The listing builds one solid part. Answer for the finished solid, in the listing's coordinates (mm). Face numbers are marked on the shaded views. A direction names the side the tool comes from. Coordinates: 2 decimals unless noted, no trailing zeros. Loops run counter-clockwise (first coordinate to the right, second up) from the corner with the lowest first, then second, coordinate; pieces in that order, holes last. Notation, with made-up numbers: M -22.5,18.5 L -13.5,18.5 A11 cw -13.5,33.5 Z; hole C 88,-37.75 d8. An arc over 180 degrees is marked long. Answer as CSV lines item,"result". Start each with the question number.
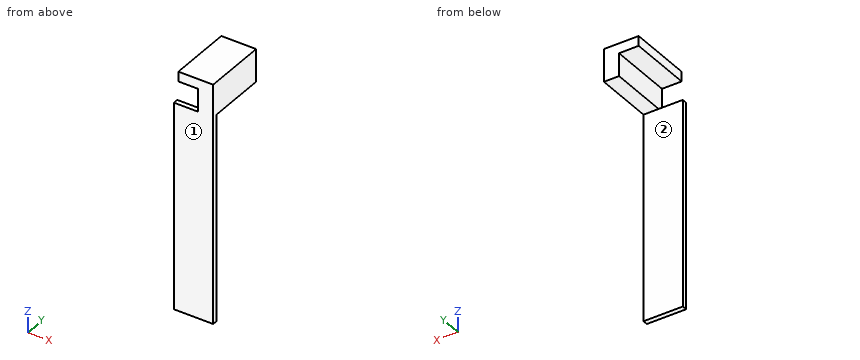
```python
from build123d import *

# Parameters (mm, degrees)
SCHIZZO1_W                   = 8
SCHIZZO1_H                   = 42.07
ESTRUSIONE_ESTRUSIONE1_DEPTH = 1
SCHIZZO2_W                   = 3.084803914
SCHIZZO2_H                   = 1
ESTRUSIONE_ESTRUSIONE2_DEPTH = 4.66
SCHIZZO3_W                   = 3.084803914
SCHIZZO3_H                   = 1
ESTRUSIONE_ESTRUSIONE3_DEPTH = 2
SCHIZZO4_W                   = 2.003143521
SCHIZZO4_H                   = 1
ESTRUSIONE_ESTRUSIONE4_DEPTH = 4
SCHIZZO5_W                   = 7.084803914
SCHIZZO5_H                   = 2.003143521
ESTRUSIONE_ESTRUSIONE5_DEPTH = 12
SCHIZZO7_W                   = 3.084803914
SCHIZZO7_H                   = 4.656856479
ESTRUSIONE_ESTRUSIONE7_DEPTH = 12


with BuildPart() as part:
    # Schizzo1 → Estrusione-Estrusione1 (new body)
    with BuildSketch(Plane(origin=(0, 0, 0), x_dir=(1, 0, 0), z_dir=(0, 1, 0))):
        with Locations((4, 21.035)):
            Rectangle(SCHIZZO1_W, SCHIZZO1_H)
    extrude(amount=ESTRUSIONE_ESTRUSIONE1_DEPTH)

    # Schizzo2 → Estrusione-Estrusione2 (add)
    with BuildSketch(Plane.XY):
        with Locations((6.457598043, 0.5)):
            Rectangle(SCHIZZO2_W, SCHIZZO2_H)
    extrude(amount=ESTRUSIONE_ESTRUSIONE2_DEPTH)

    # Schizzo3 → Estrusione-Estrusione3 (add)
    with BuildSketch(Plane.XY.offset(4.66)):
        with Locations((6.457598043, 0.5)):
            Rectangle(SCHIZZO3_W, SCHIZZO3_H)
    extrude(amount=ESTRUSIONE_ESTRUSIONE3_DEPTH)

    # Schizzo4 → Estrusione-Estrusione4 (add)
    with BuildSketch(Plane.ZY.offset(-4.915196086)):
        with Locations((5.65842824, 0.5)):
            Rectangle(SCHIZZO4_W, SCHIZZO4_H)
    extrude(amount=ESTRUSIONE_ESTRUSIONE4_DEPTH)

    # Schizzo5 → Estrusione-Estrusione5 (add)
    with BuildSketch(Plane(origin=(0, 1, 0), x_dir=(1, 0, 0), z_dir=(0, 1, 0))):
        with Locations((4.457598043, -5.65842824)):
            Rectangle(SCHIZZO5_W, SCHIZZO5_H)
    extrude(amount=ESTRUSIONE_ESTRUSIONE5_DEPTH)

    # Schizzo7 → Estrusione-Estrusione7 (add)
    with BuildSketch(Plane(origin=(0, 1, 0), x_dir=(1, 0, 0), z_dir=(0, 1, 0))):
        with Locations((6.457598043, -2.328428239)):
            Rectangle(SCHIZZO7_W, SCHIZZO7_H)
    extrude(amount=ESTRUSIONE_ESTRUSIONE7_DEPTH)


solid = part.part
```
Item 1: Section B-B on y = 10.5 is taken. Determine the outline of the cut face in (x, z).
Item 2: Section D-D on z = -33 is taken. Determine the outline of the cut face in (x, y), then the cut area to 3 significant figures.
Item 3: Each of these flat-tipped pins is pushed along its axis until it touches: P1, Ø1.2, axis at x = 2.5, y = 9, coming from the -Z side; P2, Ø1, axis at y = 7, z = 6, coming from the -X side; P3, Ø1, axis at x = 2.5, z = -21.5, coming from the +Y side; P4, Ø2, axis at x = 5.5, z = -37, coming from the -Y side. Where does it stop, or does it pass through?
Item 4: Section A-A on x = 1.75 is taken. Determine the outline of the cut face in (y, z), then the cut area to 3 significant figures.
Item 5: Section C-C on x = 7 is taken. Determine the outline of the cut face in (y, z), then the cut area to 3 significant figures.
Item 6: For the marked faces 1 and 2, determine the directions among +Z, -Z, +X, -X, +Y, -Y from which every point of the face is accessible in a straight line to the end or side of a thin tool.
Item 7: Consider line 1 (Y direction, x = 5.25, z = -8); line 2 (Z direction, x = 6.75, y = 8.5); line 3 (Z direction, x = 2.5, y = 4.5). Determine where each line is inside the solid, lowest interval first.
Results are:
1,outline,"M 0.92,4.66 L 4.92,4.66 L 4.92,0 L 8,0 L 8,6.66 L 0.92,6.66 Z"
2,outline,"M 0,0 L 8,0 L 8,1 L 0,1 Z"
2,area,"8.00 mm²"
3,P1,"z = 4.66"
3,P2,"x = 0.92"
3,P3,"y = 1"
3,P4,"y = 0"
4,outline,"M 0,-42.07 L 1,-42.07 L 1,0 L 0,0 Z; M 0,4.66 L 13,4.66 L 13,6.66 L 0,6.66 Z"
4,area,"68.1 mm²"
5,outline,"M 0,-42.07 L 1,-42.07 L 1,0 L 13,0 L 13,6.66 L 0,6.66 Z"
5,area,"129 mm²"
6,face 1,"+Z, -Z, +X, -X, -Y"
6,face 2,"-Z, +X, -X, +Y"
7,line 1,"0 to 1"
7,line 2,"0 to 6.66"
7,line 3,"4.66 to 6.66"
